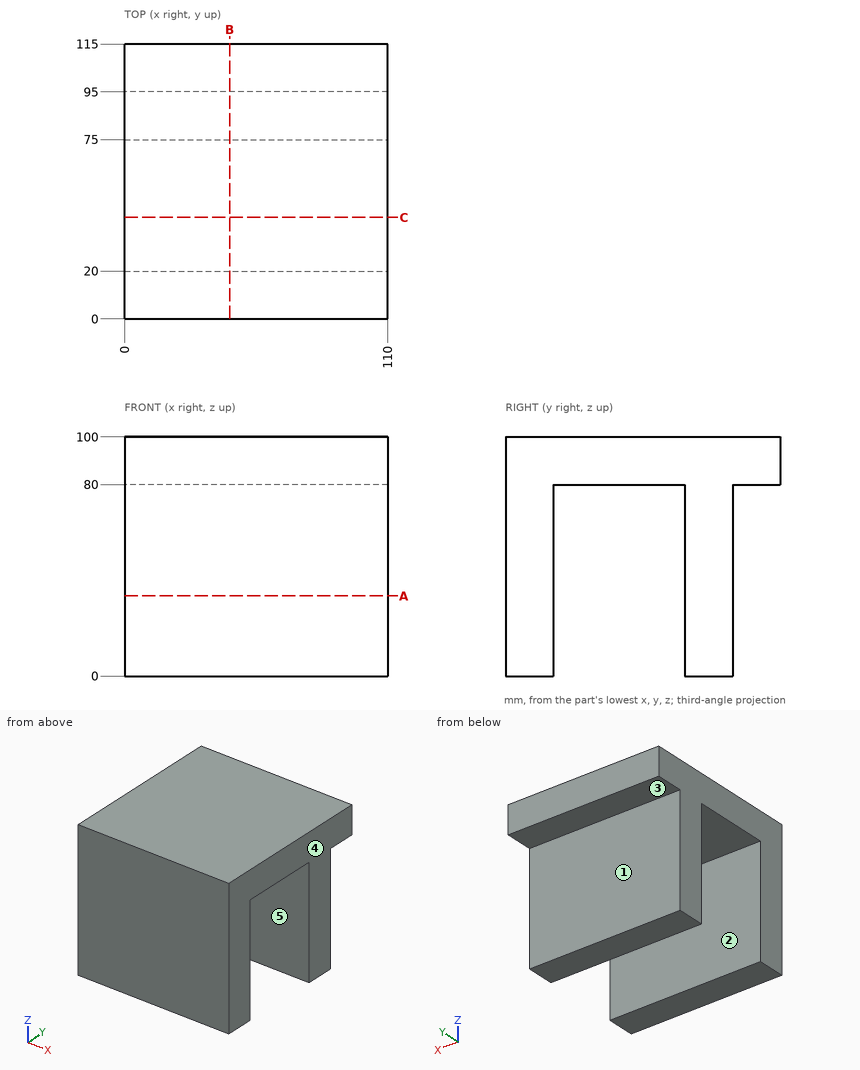
Here's the drawing with two shaded views (mm, measured from the low corner). I have some questions. A direction names the side the tool comes from. Round coordinates to 2 decimals unless told otherwise and drop trailing zeros. Write each loop counter-clockwise with the first axis right and the second up, starting at its lowest first coordinate (ties: lowest second). Pieces come first, ordered by that corner, then holes. Notation, with made-up numbers: M 84.25,22 L 113.25,22 A15 cw 113.25,26 Z; hole C -29,25 d5. An arc over 180 degrees is marked long. Answer in a Markdown table with one row per item. Add a question column.
Q1. Imagine slicing it at A-A (z = 33.5). Please give me the cut outline in (x, y), then the cut area to 3 significant figures.
Q2. Imagine slicing it at B-B (x = 44). Please give me the cut outline in (y, z).
Q3. Imagine slicing it at C-C (y = 42.5). Please give me the cut outline in (x, z).
Q4. On a 3-axis mill with a long thin cutter (end or side, diameter ignored), from which of +Z, -Z, +X, -X, +Y, -Y can I reach the whole of each face in a straight line? I mean the marked faces 4 and 5. Say none if no direction works.
Q5. Will these pins go through, and if not, where does the flat tip stop? pin 1 Ø6 at (y, z) = (71, 67) entering from -X; pin 2 Ø16 at (x, y) = (56.5, 107) entering from -Z; pin 3 Ø1.5 at (x, z) = (52.5, 41) entering from +Y.
Q6. If I drill on line 1 (Y direction, x = 10.5, z = 57.5); line 2 (Z direction, x = 78, y = 31.5), over which ranges is the centre line in solid material (lowest first)? Write a range as from..to.
Q7. If we mould it in two halves opening along Y, with no side actions, what happens to the marked faces 1, 2 and 3? For each: +Y half, -Y half, draft (parallel to the pull), parting line (faces both ways), or undercut.
Values:
| question | item | result |
|---|---|---|
| 1 | outline | M 0,0 L 110,0 L 110,20 L 0,20 Z; M 0,75 L 110,75 L 110,95 L 0,95 Z |
| 1 | area | 4,400 mm^2 |
| 2 | outline | M 0,0 L 20,0 L 20,80 L 75,80 L 75,0 L 95,0 L 95,80 L 115,80 L 115,100 L 0,100 Z |
| 3 | outline | M 0,80 L 110,80 L 110,100 L 0,100 Z |
| 4 | face 4 | +Z, -Z, +X, +Y, -Y |
| 4 | face 5 | -Z, +X, -X |
| 5 | pin 1 | through |
| 5 | pin 2 | z = 80 |
| 5 | pin 3 | y = 95 |
| 6 | line 1 | 0..20, 75..95 |
| 6 | line 2 | 80..100 |
| 7 | face 1 | +Y half |
| 7 | face 2 | undercut |
| 7 | face 3 | draft |
